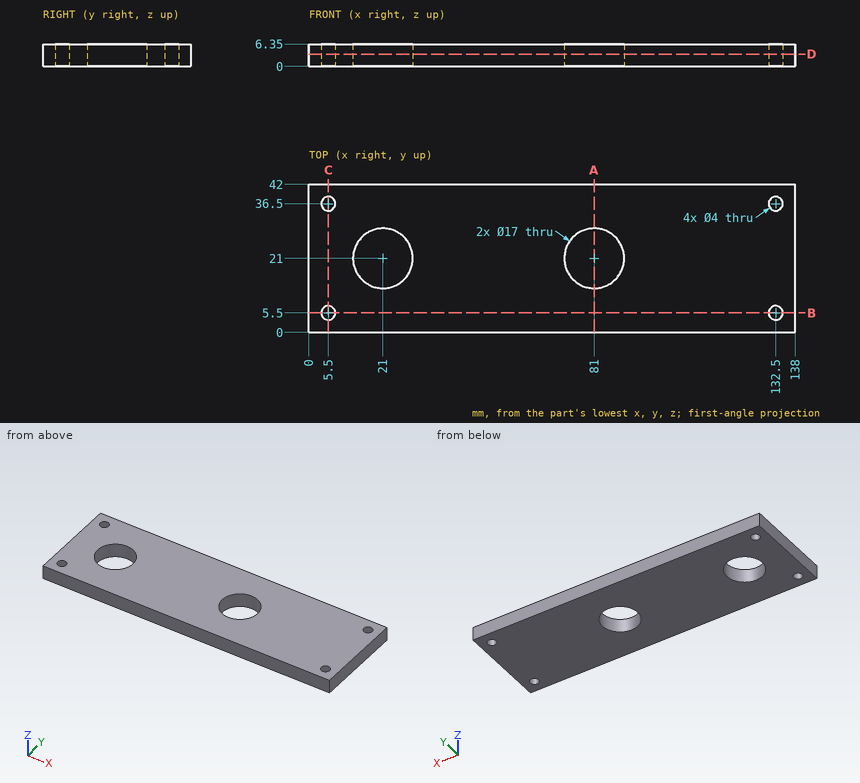
Geometry check sheet. Reference: drawing and pictorial views, mm from the part's lowest x, y, z. Round coordinates to 2 decimals unless told otherwise and drop trailing zeros. Order: outer loops, then holes, each group sorted by start corner. A loop starts at its lowest first (then second) coordinate and runs counter-clockwise, first axis right, second up. Notation, with made-up numbers: (72, 79) - (88, 79) arc R12 cw to (88, 90) - close; hole circle Ø4 at (10, 66.25). An arc over 180 degrees is marked (long way). Use a Markdown table: item, result. Add a question column.
1) Section check A-A (x = 81). Record the cut outline in (y, z), then the cut area to 3 significant figures.
2) Section check D-D (z = 3.5). Record the cut outline in (x, y).
3) Section check C-C (x = 5.5). Record the cut outline in (y, z), then the cut area to 3 significant figures.
4) Thickness scan on line 1 along Y through (x, z) = (5.5, 4.5); line 2 along X through (y, z) = (35.5, 4.75); line 3 along Y through (x, z) = (21, 4.5). Record the ranges inside material, lowest first.
5) Section check B-B (y = 5.5). Record the cut outline in (x, z).
Established:
| question | item | result |
|---|---|---|
| 1 | outline | (0, 0) - (12.5, 0) - (12.5, 6.35) - (0, 6.35) - close; (29.5, 0) - (42, 0) - (42, 6.35) - (29.5, 6.35) - close |
| 1 | area | 159 mm2 |
| 2 | outline | (0, 0) - (138, 0) - (138, 42) - (0, 42) - close; hole circle Ø4 at (5.5, 5.5); hole circle Ø4 at (5.5, 36.5); hole circle Ø17 at (21, 21); hole circle Ø17 at (81, 21); hole circle Ø4 at (132.5, 5.5); hole circle Ø4 at (132.5, 36.5) |
| 3 | outline | (0, 0) - (3.5, 0) - (3.5, 6.35) - (0, 6.35) - close; (7.5, 0) - (34.5, 0) - (34.5, 6.35) - (7.5, 6.35) - close; (38.5, 0) - (42, 0) - (42, 6.35) - (38.5, 6.35) - close |
| 3 | area | 216 mm2 |
| 4 | line 1 | 0 to 3.5, 7.5 to 34.5, 38.5 to 42 |
| 4 | line 2 | 0 to 3.77, 7.23 to 130.77, 134.23 to 138 |
| 4 | line 3 | 0 to 12.5, 29.5 to 42 |
| 5 | outline | (0, 0) - (3.5, 0) - (3.5, 6.35) - (0, 6.35) - close; (7.5, 0) - (130.5, 0) - (130.5, 6.35) - (7.5, 6.35) - close; (134.5, 0) - (138, 0) - (138, 6.35) - (134.5, 6.35) - close |
